The listing builds one solid part. Answer for the finished solid, in the listing's coordinates (mm). A direction names the side the tool comes from. Coordinates: 2 decimals unless noted, no trailing zeros. Order: outer loops, then holes, each group sorted by start corner. A loop starts at its lowest first (then second) coordinate and runs counter-clockwise, first axis right, second up.
Autodesk Inventor part; units mm, degrees
ref_plane "YZ Plane" through (0, 0, 0) normal (1, 0, 0) x (0, 1, 0)
ref_plane "XZ Plane" through (0, 0, 0) normal (0, 1, 0) x (-1, 0, 0)
ref_plane "XY Plane" through (0, 0, 0) normal (0, 0, 1) x (1, 0, 0)
sketch "Sketch1" plane through (0, 0, 0) normal (0, 1, 0) x (-1, 0, 0)
  line L0 (0, -2) -> (0, -108)
  line L1 (2, -110) -> (63, -110)
  line L2 (2, 0) -> (63, 0)
  line L3 (65, -2) -> (65, -108)
  line L4 (0, 0) -> (0, -3)
  line L5 (65, 0) -> (57, 0)
  line L6 (0, -110) -> (0, -107)
  line L7 (0, 0) -> (3, 0)
  arc A0 (65, -2) -> (63, 0) centre (63, -2) ccw
  arc A1 (2, 0) -> (0, -2) centre (2, -2) ccw
  arc A2 (0, -108) -> (2, -110) centre (2, -108) ccw
  arc A3 (63, -110) -> (65, -108) centre (63, -108) ccw
  arc A4 (5, -3) -> (3, -5) centre (5, -5) ccw
  circle A5 centre (7, -7) radius 1.5
  line L8 (11, -3) -> (11, -9)
  line L9 (9, -11) -> (3, -11)
  arc A6 (9, -11) -> (11, -9) centre (9, -9) ccw
  line L10 (3, -5) -> (3, -11)
  arc A7 (3, -105) -> (5, -107) centre (5, -105) ccw
  circle A8 centre (7, -103) radius 1.5
  line L11 (11, -107) -> (11, -101)
  line L12 (9, -99) -> (3, -99)
  arc A9 (11, -101) -> (9, -99) centre (9, -101) ccw
  line L13 (3, -105) -> (3, -99)
  line L14 (3, -11) -> (3, -99)
  line L15 (11, -107) -> (5, -107)
  line L16 (11, -3) -> (5, -3)
  arc A10 (62, -5) -> (60, -3) centre (60, -5) ccw
  circle A11 centre (58, -7) radius 1.5
  line L17 (54, -3) -> (54, -9)
  line L18 (56, -11) -> (62, -11)
  arc A12 (54, -9) -> (56, -11) centre (56, -9) ccw
  line L19 (62, -5) -> (62, -11)
  arc A13 (56, -99) -> (54, -101) centre (56, -101) ccw
  circle A14 centre (58, -103) radius 1.5
  line L20 (56, -99) -> (62, -99)
  line L21 (62, -105) -> (62, -99)
  arc A15 (60, -107) -> (62, -105) centre (60, -105) ccw
  line L22 (54, -107) -> (54, -101)
  line L23 (62, -11) -> (62, -99)
  line L24 (54, -107) -> (60, -107)
  line L25 (54, -3) -> (60, -3)
  line L26 (54, -107) -> (11, -107)
  line L27 (54, -3) -> (11, -3)
  point P0 (65, -110)
  point P1 (55, -5)
  point P2 (55, -105)
  dimension "d0" = 110
  dimension "d1" = 65
  dimension "d2" = 3
  dimension "d4" = 3
  dimension "d5" = 3
  dimension "d8" = 2
extrude "Extrusion18" add sketch "Sketch1" along normal blind 20 contours A1 L2 A0 L3 A3 L1 A2 L0 | L16 L8 A6 L9 L10 A4 | L27 L17 A12 L18 L23 L20 A13 L22 L26 L11 A9 L12 L14 L9 A6 L8 | L25 A10 L19 L18 A12 L17 | L12 A9 L11 L15 A7 L13 | L21 A15 L24 L22 A13 L20 | A5 | A8 | A11 | A14
extrude "Extrusion19" cut sketch "Sketch1" along normal blind 18 contours L27 L17 A12 L18 L23 L20 A13 L22 L26 L11 A9 L12 L14 L9 A6 L8
extrude "Extrusion20" cut sketch "Sketch1" along normal blind 20 contours A5 | A8 | A11 | A14
extrude "Extrusion21" add sketch "Sketch1" along normal blind 21.5 contours L16 L8 A6 L9 L10 A4 | L25 A10 L19 L18 A12 L17 | L12 A9 L11 L15 A7 L13 | L21 A15 L24 L22 A13 L20
sketch "Sketch11" plane through (0, 21.5, 0) normal (0, 1, 0) x (1, 0, 0)
  circle A0 centre (-7, 7) radius 1.5
  circle A1 centre (-7, 7) radius 2.5
  circle A2 centre (-7, 103) radius 1.5
  circle A3 centre (-7, 103) radius 2.5
  circle A4 centre (-58, 103) radius 1.5
  circle A5 centre (-58, 103) radius 2.5
  circle A6 centre (-58, 7) radius 1.5
  circle A7 centre (-58, 7) radius 2.5
  point P0 (0, 0)
  dimension "d166" = 5
  dimension "d167" = 5
  dimension "d168" = 5
  dimension "d169" = 5
extrude "Extrusion22" cut sketch "Sketch11" against normal blind 1.5 contours A1 | A3 | A5 | A6 | A7
sketch "Sketch12" plane through (-65, 0, -108) normal (-1, 0, 0) x (0, 0, 1)
  line L0 (99, 0) -> (99, 18)
  line L1 (7, 0) -> (7, 18)
  line L2 (99, 0) -> (7, 0)
  line L3 (97, 0) -> (9, 0)
  line L4 (53, 2) -> (27, 2)
  line L5 (53, 2) -> (79, 2)
  line L6 (80, 1) -> (80, 0)
  line L7 (26, 1) -> (26, 0)
  line L8 (20, 10) -> (14, 10)
  line L9 (13, 11) -> (13, 11.5)
  line L10 (21, 11) -> (21, 11.5)
  line L11 (20, 12.5) -> (14, 12.5)
  arc A0 (80, 1) -> (79, 2) centre (79, 1) ccw
  arc A1 (27, 2) -> (26, 1) centre (27, 1) ccw
  arc A2 (20, 10) -> (21, 11) centre (20, 11) ccw
  arc A3 (21, 11.5) -> (20, 12.5) centre (20, 11.5) ccw
  arc A4 (14, 12.5) -> (13, 11.5) centre (14, 11.5) ccw
  arc A5 (13, 11) -> (14, 10) centre (14, 11) ccw
  point P0 (108, 0)
  point P1 (26, 2)
  point P2 (80, 2)
  point P3 (21, 10)
  point P4 (13, 10)
  point P5 (13, 12.5)
  dimension "d173" = 27
  dimension "d174" = 27
  dimension "d179" = 8
  dimension "d180" = 2.5
  dimension "d181" = 1
  dimension "d182" = 1
extrude "Extrusion23" cut sketch "Sketch12" against normal blind 3
sketch "Sketch13" plane through (0, 20, 0) normal (0, 1, 0) x (1, 0, 0)
  line L0 (-62, 11) -> (-56, 11)
  line L1 (-3, 99) -> (-9, 99)
  line L2 (-62, 99) -> (-3, 99)
  line L3 (-3, 11) -> (-3, 99)
  line L4 (-3, 99) -> (-3, 11)
  line L5 (-3, 11) -> (-62, 11)
  line L6 (-62, 55) -> (-3, 55)
  line L7 (-62, 55) -> (-62, 11)
  line L8 (-62, 29) -> (-62, 81)
  line L9 (-3, 55) -> (-62, 55)
  line L10 (-37.5, 34.5) -> (-59.5, 34.5)
  line L11 (-59.5, 34.5) -> (-59.5, 31.5)
  line L12 (-59.5, 31.5) -> (-37.5, 31.5)
  line L13 (-37.5, 31.5) -> (-37.5, 34.5)
  line L14 (-27.5, 34.5) -> (-5.5, 34.5)
  line L15 (-5.5, 34.5) -> (-5.5, 31.5)
  line L16 (-5.5, 31.5) -> (-27.5, 31.5)
  line L17 (-27.5, 31.5) -> (-27.5, 34.5)
  line L18 (-37.5, 75.5) -> (-59.5, 75.5)
  line L19 (-59.5, 75.5) -> (-59.5, 78.5)
  line L20 (-59.5, 78.5) -> (-37.5, 78.5)
  line L21 (-37.5, 78.5) -> (-37.5, 75.5)
  line L22 (-27.5, 75.5) -> (-5.5, 75.5)
  line L23 (-5.5, 75.5) -> (-5.5, 78.5)
  line L24 (-5.5, 78.5) -> (-27.5, 78.5)
  line L25 (-27.5, 78.5) -> (-27.5, 75.5)
  point P0 (0, 0)
  dimension "d202" = 22
  dimension "d203" = 3
extrude "Extrusion24" cut sketch "Sketch13" against normal blind 3 contours L13 L12 L11 L10 | L14 L15 L16 L17 | L18 L19 L20 L21 | L25 L24 L23 L22
sketch "Sketch14" plane through (-2, 0, -110) normal (0, 0, -1) x (-1, 0, 0)
  line L0 (0, 0) -> (61, 0)
  line L1 (7, 0) -> (7, 18)
  line L2 (13.5993, 5.8762) -> (13.5993, 13.8762)
  line L3 (14.5993, 14.8762) -> (32.5993, 14.8762)
  line L4 (33.5993, 13.8762) -> (33.5993, 5.8762)
  line L5 (32.5993, 4.8762) -> (14.5993, 4.8762)
  arc A0 (32.5993, 4.8762) -> (33.5993, 5.8762) centre (32.5993, 5.8762) ccw
  arc A1 (13.5993, 5.8762) -> (14.5993, 4.8762) centre (14.5993, 5.8762) ccw
  arc A2 (14.5993, 14.8762) -> (13.5993, 13.8762) centre (14.5993, 13.8762) ccw
  arc A3 (33.5993, 13.8762) -> (32.5993, 14.8762) centre (32.5993, 13.8762) ccw
  point P0 (-2, 0)
  point P1 (13.5993, 4.8762)
  point P2 (13.5993, 14.8762)
  point P3 (33.5993, 14.8762)
  dimension "d194" = 10
  dimension "d195" = 20
  dimension "d196" = 1
extrude "Extrusion25" cut sketch "Sketch14" against normal blind 3
properties part number "Part 2 edit"
(1) Find section D-D (z = -67.5). Write down the section's boundary in (x, y).
(2) The mould has two halves that part along Z. Classify faces 1 (the face through (-58.33, 20.76, -105.48)), 2 (the face through (-35.599, 10, -109)), 3 (the face through (-0.6, 9.86, -109.43)): released by +Z, released by -Z, zero draft, split by the parting line, or undercut.
(3) Find section C-C (x = -48.5). Write down the section's boundary in (y, z).
(4) Each of these flat-tipped pins is pushed along its axis until it touches: pin 1 Ø3 at (x, z) = (-11.5, -57) entering from -Y; pin 2 Ø1.6 at (x, y) = (-6, 21) entering from +Z; pin 3 Ø2.5 at (x, z) = (-63, -63.5) entering from -Y; pin 4 Ø2.5 at (x, z) = (-58, -7) entering from +Y. Where does it stop, or does it pass through?
(5) For faces 4 (the face through (-27.5, 19, -33)), 5 (the face through (-32, 18, -54)), 6 (the face through (-3.57, 20.74, -3.6)), determine the directions among +Z, -Z, +X, -X, +Y, -Y from which every point of the face is accessible in a straight line to the end or side of a thin tool.
(6) Consider line 1 (X direction, y = 9, z = -103); line 2 (Z direction, x = -54.5, y = 18.75); line 3 (X direction, y = 21.05, z = -7). Determine where each line is inside the solid, lowest interval first.
(7) Find section B-B (z = -7). Give the number of separate pieces and of enclosed holes in the cut face, and give its area (3 significant figures).
(8) Find section A-A (y = 16). Write down the section's boundary in (x, z).
Findings below:
1. outline: (-65, 2) - (-62, 2) - (-62, 18) - (-3, 18) - (-3, 0) - (0, 0) - (0, 20) - (-65, 20) - close
2. face 1: undercut
2. face 2: zero draft
2. face 3: released by -Z
3. outline: (0, -110) - (20, -110) - (20, -78.5) - (18, -78.5) - (18, -107) - (0, -107) - close; (0, -3) - (18, -3) - (18, -31.5) - (20, -31.5) - (20, 0) - (0, 0) - close; (18, -75.5) - (20, -75.5) - (20, -34.5) - (18, -34.5) - close
4. pin 1: stops at y = 18
4. pin 2: stops at z = -3
4. pin 3: stops at y = 2
4. pin 4: passes through
5. face 4: +Y, -Y
5. face 5: -Y
5. face 6: +Z, +X, +Y
6. line 1: x = -65 to -59.5, -56.5 to -54, -11 to -8.5, -5.5 to 0
6. line 2: z = -110 to -78.5, -75.5 to -34.5, -31.5 to 0
6. line 3: x = -62 to -60.5, -55.5 to -54, -11 to -9.5, -4.5 to -3
7. separate pieces: 3
7. enclosed holes: 0
7. area: 415 mm2
8. outline: (-65, -108) arc R2 ccw to (-63, -110) - (-2, -110) arc R2 ccw to (0, -108) - (0, -2) arc R2 ccw to (-2, 0) - (-63, 0) arc R2 ccw to (-65, -2) - close; hole (-62, -99) - (-56, -99) arc R2 cw to (-54, -101) - (-54, -107) - (-11, -107) - (-11, -101) arc R2 cw to (-9, -99) - (-3, -99) - (-3, -11) - (-9, -11) arc R2 cw to (-11, -9) - (-11, -3) - (-54, -3) - (-54, -9) arc R2 cw to (-56, -11) - (-62, -11) - close; hole circle Ø3 at (-58, -103); hole circle Ø3 at (-58, -7); hole circle Ø3 at (-7, -103); hole circle Ø3 at (-7, -7)
